Design review of the part built by this model. Coordinates are the model's own, in mm. A direction names the side the tool comes from. Coordinates: 2 decimals unless noted, no trailing zeros. Order: outer loops, then holes, each group sorted by start corner. A loop starts at its lowest first (then second) coordinate and runs counter-clockwise, first axis right, second up.
from build123d import *

# Parameters (mm, degrees)
SKETCH1_R           = 9.525
SKETCH1_R_2         = 4
BOSS_EXTRUDE1_DEPTH = 38.1
FILLET1_R           = 19.05
SKETCH2_W           = 24.13
SKETCH2_H           = 38.1
CUT_EXTRUDE1_DEPTH  = 254.443765952
CUT_EXTRUDE2_DEPTH  = 12.7
SKETCH4_R           = 3
CUT_EXTRUDE3_DEPTH  = 254.443765952
FILLET4_R           = 5
FILLET5_R           = 5


# Some blends are built 0.0001 mm under size
with BuildPart() as part:
    # Sketch1 → Boss-Extrude1 (new body)
    with BuildSketch(Plane(origin=(0, 0, 0), x_dir=(0, 0, -1), z_dir=(1, 0, 0))):
        with BuildLine():
            ThreePointArc((9.682458366, 16.55), (0, 9.05), (-9.682458366, 16.55))
            Line((-9.682458366, 16.55), (-25, 16.55))
            Line((-25, 16.55), (-25, 0))
            Line((-25, 0), (247.65, 0))
            Line((247.65, 0), (247.65, 38.1))
            Line((247.65, 38.1), (-25, 38.1))
            Line((-25, 38.1), (-25, 21.55))
            Line((-25, 21.55), (-9.682458366, 21.55))
            ThreePointArc((-9.682458366, 21.55), (0, 29.05), (9.682458366, 21.55))
            Line((9.682458366, 21.55), (15, 21.55))
            Line((15, 21.55), (15, 16.55))
            Line((15, 16.55), (9.682458366, 16.55))
        make_face()
        with Locations(Location((139.7, 19.05, 0), (0, 0, 180))):
            Circle(SKETCH1_R, mode=Mode.SUBTRACT)
        with Locations(Location((228.6, 19.05, 0), (0, 0, 180))):
            Circle(SKETCH1_R_2, mode=Mode.SUBTRACT)
    extrude(amount=BOSS_EXTRUDE1_DEPTH)

    # Fillet1
    fillet1_edges = [part.edges().sort_by_distance(p)[0] for p in [
        (19.05, 0, -247.65),
        (19.05, 38.1, -247.65),
    ]]
    fillet(fillet1_edges, radius=FILLET1_R - 0.0001)  # a hair under: the kernel refuses the full size

    # Sketch2 → Cut-Extrude1 (cut, through all)
    with BuildSketch(Plane(origin=(0, 38.1, 0), x_dir=(1, 0, 0), z_dir=(0, 1, 0))):
        with Locations((19.05, 228.6)):
            Rectangle(SKETCH2_W, SKETCH2_H)
    extrude(amount=-CUT_EXTRUDE1_DEPTH, mode=Mode.SUBTRACT)

    # Sketch3 → Cut-Extrude2 (cut)
    with BuildSketch(Plane(origin=(38.1, 0, 0), x_dir=(0, 0, -1), z_dir=(1, 0, 0))):
        with BuildLine():
            Line((34.7, 5.08), (109.7, 5.08))
            ThreePointArc((109.7, 5.08), (123.67, 19.05), (109.7, 33.02))
            Line((109.7, 33.02), (34.7, 33.02))
            ThreePointArc((34.7, 33.02), (20.73, 19.05), (34.7, 5.08))
        make_face()
        with BuildLine():
            Line((169.7, 5.08), (193.9, 5.08))
            ThreePointArc((193.9, 5.08), (207.87, 19.05), (193.9, 33.02))
            Line((193.9, 33.02), (169.7, 33.02))
            ThreePointArc((169.7, 33.02), (155.73, 19.05), (169.7, 5.08))
        make_face()
        with BuildLine():
            ThreePointArc((31.430916309, 19.05), (30.759207099, 25.513256042), (28.772789625, 31.700259965))
            ThreePointArc((28.772789625, 31.700259965), (20.73, 19.05), (28.772789625, 6.399740035))
            ThreePointArc((28.772789625, 6.399740035), (30.759207099, 12.586743958), (31.430916309, 19.05))
        make_face()
    cut_extrude2 = extrude(amount=-CUT_EXTRUDE2_DEPTH, mode=Mode.SUBTRACT)

    # Mirror1: Cut-Extrude2 across plane
    add(cut_extrude2.mirror(Plane(origin=(19.05, 0, 0), x_dir=(0, 0, 1), z_dir=(1, 0, 0))), mode=Mode.SUBTRACT)

    # Sketch4 → Cut-Extrude3 (cut, through all)
    with BuildSketch(Plane(origin=(0, 38.1, 0), x_dir=(1, 0, 0), z_dir=(0, 1, 0))):
        with Locations(Location((7.5, -17.5, 0), (0, 0, 270))):
            Circle(SKETCH4_R)
        with Locations(Location((30.6, -17.5, 0), (0, 0, 270))):
            Circle(SKETCH4_R)
    extrude(amount=-CUT_EXTRUDE3_DEPTH, mode=Mode.SUBTRACT)

    # Fillet4
    fillet4_edges = [part.edges().sort_by_distance(p)[0] for p in [
        (19.05, 38.1, -209.55),
        (19.05, 0, -209.55),
    ]]
    fillet(fillet4_edges, radius=FILLET4_R)

    # Fillet5
    # the kernel refuses this fillet: 5 mm, written as the material it adds along each edge
    with BuildSketch(Plane(origin=(31.115, 33.1, -209.55), x_dir=(-1, 0, 0), z_dir=(0, -1, 0))) as fillet5_piece_1:
        with BuildLine():
            CenterArc((FILLET5_R, FILLET5_R), FILLET5_R, 180, 90)
            Line((0, FILLET5_R), (0, 0))
            Line((0, 0), (FILLET5_R, 0))
        make_face()
    extrude(amount=28.1)
    with BuildSketch(Plane(origin=(6.985, 33.1, -209.55), x_dir=(1, 0, 0), z_dir=(0, -1, 0))) as fillet5_piece_2:
        with BuildLine():
            CenterArc((FILLET5_R, -FILLET5_R), FILLET5_R, 90, 90)
            Line((0, -FILLET5_R), (0, 0))
            Line((0, 0), (FILLET5_R, 0))
        make_face()
    extrude(amount=28.1)
    with BuildSketch(Plane(origin=(31.115, 5, -204.55), x_dir=(0, 0.8017442392976496, 0.597667277632826), z_dir=(0, 0.597667277632826, -0.8017442392976496))) as fillet5_piece_3_section:
        with BuildLine():
            CenterArc((5 + FILLET5_R, -FILLET5_R), FILLET5_R, 90, 90)
            Line((5 + FILLET5_R, 0), (5, 0))
            Line((5, 0), (5, -FILLET5_R))
        make_face()
    fillet5_piece_3 = revolve(axis=Axis((31.115, 5, -204.55), (1, 0, 0)), revolution_arc=233.296989237, mode=Mode.PRIVATE)
    fillet5_piece_3 = split(fillet5_piece_3, bisect_by=Plane(origin=(29.55685837, 0, -208.299694711), z_dir=(0, 1, 0)), keep=Keep.TOP, mode=Mode.PRIVATE)
    fillet5_piece_3 = fillet5_piece_3 - Plane(origin=(29.55685837, 19.05, -193.9), x_dir=(0, -1, 0), z_dir=(1, 0, 0)) * Cylinder(13.97, 41, mode=Mode.PRIVATE)
    add(fillet5_piece_3)
    with BuildSketch(Plane(origin=(6.985, 5, -204.55), x_dir=(0, 0.8017442392976496, 0.597667277632826), z_dir=(0, 0.597667277632826, -0.8017442392976496))) as fillet5_piece_4_section:
        with BuildLine():
            CenterArc((5 + FILLET5_R, FILLET5_R), FILLET5_R, 180, 90)
            Line((5, FILLET5_R), (5, 0))
            Line((5, 0), (5 + FILLET5_R, 0))
        make_face()
    fillet5_piece_4 = revolve(axis=Axis((6.985, 5, -204.55), (1, 0, 0)), revolution_arc=233.296989237, mode=Mode.PRIVATE)
    fillet5_piece_4 = split(fillet5_piece_4, bisect_by=Plane(origin=(8.543141587, 0, -208.299694664), z_dir=(0, 1, 0)), keep=Keep.TOP, mode=Mode.PRIVATE)
    fillet5_piece_4 = fillet5_piece_4 - Plane(origin=(8.543141587, 19.05, -193.9), x_dir=(0, -1, 0), z_dir=(-1, 0, 0)) * Cylinder(13.97, 41, mode=Mode.PRIVATE)
    add(fillet5_piece_4)
    with BuildSketch(Plane(origin=(31.115, 33.1, -204.55), x_dir=(0, 0, -1), z_dir=(0, -1, 0))) as fillet5_piece_5_section:
        with BuildLine():
            CenterArc((5 + FILLET5_R, -FILLET5_R), FILLET5_R, 90, 90)
            Line((5 + FILLET5_R, 0), (5, 0))
            Line((5, 0), (5, -FILLET5_R))
        make_face()
    fillet5_piece_5 = revolve(axis=Axis((31.115, 33.1, -204.55), (1, 0, 0)), revolution_arc=233.296989237, mode=Mode.PRIVATE)
    fillet5_piece_5 = split(fillet5_piece_5, bisect_by=Plane(origin=(29.556858367, 38.1, -208.299694701), z_dir=(0, -1, 0)), keep=Keep.TOP, mode=Mode.PRIVATE)
    fillet5_piece_5 = fillet5_piece_5 - Plane(origin=(29.556858367, 19.05, -193.9), x_dir=(0, -1, 0), z_dir=(1, 0, 0)) * Cylinder(13.97, 40, mode=Mode.PRIVATE)
    add(fillet5_piece_5)
    with BuildSketch(Plane(origin=(6.985, 33.1, -204.55), x_dir=(0, 0, -1), z_dir=(0, -1, 0))) as fillet5_piece_6_section:
        with BuildLine():
            CenterArc((5 + FILLET5_R, FILLET5_R), FILLET5_R, 180, 90)
            Line((5 + FILLET5_R, 0), (5, 0))
            Line((5, 0), (5, FILLET5_R))
        make_face()
    fillet5_piece_6 = revolve(axis=Axis((6.985, 33.1, -204.55), (1, 0, 0)), revolution_arc=233.296989237, mode=Mode.PRIVATE)
    fillet5_piece_6 = split(fillet5_piece_6, bisect_by=Plane(origin=(8.54314159, 38.1, -208.299694655), z_dir=(0, -1, 0)), keep=Keep.TOP, mode=Mode.PRIVATE)
    fillet5_piece_6 = fillet5_piece_6 - Plane(origin=(8.54314159, 19.05, -193.9), x_dir=(0, -1, 0), z_dir=(-1, 0, 0)) * Cylinder(13.97, 40, mode=Mode.PRIVATE)
    add(fillet5_piece_6)


solid = part.part
1. To check wall thickness, follow line 1 (X direction, y = 34, z = 17); line 2 (Z direction, x = 35, y = 19); line 3 (Y direction, x = 11.5, z = -139.7) (3 decimals). State the ranges of each line that lie inside material, in increasing order.
2. Add section D-D (z = -57.5). Give the boundary of the cut face in (x, y).
3. Add section B-B (x = 15.5). Give the boundary of the cut face in (y, z) (3 decimals).
4. Add section A-A (z = 17.5). Give the boundary of the cut face in (x, y).
5. Add section C-C (y = 12). State how many separate pieces and enclosed holes the cut face has, and give its area (3 significant figures).
6. For faces 1 (the flat face through (25.4, 19, -181)), 2 (the cylindrical face through (19.15, 36.6, -208.12)), 3 (the flat face through (19, 21.55, -12)), 4 (the flat face through (6, 5.08, -182)), 5 (the flat face through (19, 19, -209.55)), list the 3-axis set-ups (+Z, -Z, +X, -X, +Y, -Y) from which the entire face can be reached by the end or side of a thin tool; tool diameter is ignored.
7. Mouldability with a two-part tool opening along Y and no side actions: class faces 6 (the flat face through (25.4, 19, -71)), 7 (the cylindrical face through (19.15, 1.43, -208.05)), 8 (the flat face through (0, 36, -109)) as pulls with the +Y half, pulls with the -Y half, needs draft (parallel to the pull), parting line crosses it, or undercut.
8. Insertion check: pin 1 (6 mm diameter, centred on x = 22.5, z = -12, fed in from -Y); pin 2 (11.5 mm diameter, centred on x = 19.5, y = 21.5, fed in from -Z); pin 3 (14 mm diameter, centred on y = 16.5, z = -186, fed in from -X); pin 4 (3.5 mm diameter, centred on x = 7.5, z = 17.5, fed in from -Y). Each pin has a flat end and moves straight along its axis. Give the tip position at first contact, or say it passes through.
Solution:
1. line 1: x = 0 to 4.54, 10.46 to 27.64, 33.56 to 38.1
1. line 2: z = -247.65 to -232.6, -224.6 to -207.87, -155.73 to -149.22, -130.18 to -123.67, -20.73 to -15
1. line 3: y = 0 to 9.525, 28.575 to 38.1
2. outline: (0, 0) - (38.1, 0) - (38.1, 5.08) - (25.4, 5.08) - (25.4, 33.02) - (38.1, 33.02) - (38.1, 38.1) - (0, 38.1) - (0, 33.02) - (12.7, 33.02) - (12.7, 5.08) - (0, 5.08) - close
3. outline: (0, -204.55) arc R5 ccw to (5, -209.55) - (33.1, -209.55) arc R5 ccw to (38.1, -204.55) - (38.1, 25) - (21.55, 25) - (21.55, 9.682) arc R10 cw to (21.55, -9.682) - (21.55, -15) - (16.55, -15) - (16.55, -9.682) arc R10 cw to (16.55, 9.682) - (16.55, 25) - (0, 25) - close; hole circle Ø19.05 at (19.05, -139.7)
4. outline: (0, 0) - (4.5, 0) - (4.5, 16.55) - (0, 16.55) - close; (0, 21.55) - (4.5, 21.55) - (4.5, 38.1) - (0, 38.1) - close; (10.5, 0) - (27.6, 0) - (27.6, 16.55) - (10.5, 16.55) - close; (10.5, 21.55) - (27.6, 21.55) - (27.6, 38.1) - (10.5, 38.1) - close; (33.6, 0) - (38.1, 0) - (38.1, 16.55) - (33.6, 16.55) - close; (33.6, 21.55) - (38.1, 21.55) - (38.1, 38.1) - (33.6, 38.1) - close
5. separate pieces: 3
5. enclosed holes: 2
5. area: 4,630 mm2
6. face 1: +X
6. face 2: -Z, +Y
6. face 3: +Z, +X, -X
6. face 4: -X
6. face 5: -Z, +Y, -Y
7. face 6: undercut
7. face 7: pulls with the -Y half
7. face 8: needs draft
8. pin 1: stops at y = 0
8. pin 2: stops at z = -209.55
8. pin 3: stops at x = 12.7
8. pin 4: passes through
